Source: three-view drawing plus pictorial views. Frame: mm from the lowest corner of the part. Give positions to 0.01 mm unless a question says otherwise; leave off trailing zeros. Order: outer loops, then holes, each group sorted by start corner. A loop starts at its lowest first (then second) coordinate and runs counter-clockwise, first axis right, second up.
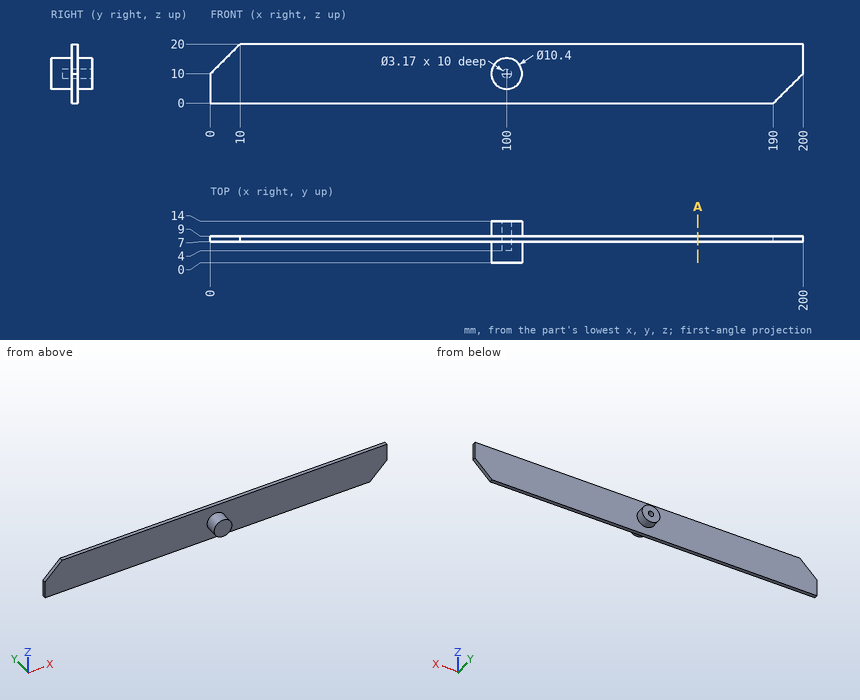
1) Ray query, L1, parallel to Z at x = 100, y = 11 (3 decimals); L2, parallel to Y at x = 150, z = 1.5; L3, parallel to X at y = 11.5, z = 11. Return the intervals inside material, ascending.
Checks:
L1: z = 4.8 to 8.415, 11.585 to 15.2
L2: y = 7 to 9
L3: x = 94.9 to 98.77, 101.23 to 105.1
2) Section query A-A on x = 164.5. Output: boundary loops of the cut face in (y, z).
Checks:
outline: (7, 0) - (9, 0) - (9, 20) - (7, 20) - close
3) First-contact query: pin 1 Ø4 at (y, z) = (9, 6.5) entering from +X; pin 2 Ø10 at (x, z) = (120, 11.5) entering from -Y; pin 3 Ø1 at (y, z) = (5, 11.5) entering from -X. Flat tips, straight axial feed; report the tip coordinate or a pass-through.
Checks:
pin 1: stops at x = 198.5
pin 2: stops at y = 7
pin 3: stops at x = 94.9
